from build123d import *

# Parameters (mm, degrees)
PAD_DEPTH       = 1.6
CHAMFER_SIZE    = 0.5
POCKET_DEPTH    = 1.601
PAD018_DEPTH    = 2.5
SKETCH028_R     = 2
POCKET006_DEPTH = 1.6
SKETCH029_R     = 1
POCKET007_DEPTH = 2.501
CHAMFER003_SIZE = 0.95


with BuildPart() as part:
    # Sketch (on Face1 of Binder) → Pad (new body)
    with BuildSketch(Plane.XZ.offset(29.45)):
        with BuildLine():
            Line((-19.5, 11.5), (19.5, 11.5))
            ThreePointArc((21.1, 9.9), (20.631371, 11.031371), (19.5, 11.5))
            Line((21.1, 9.9), (21.1, -1.6))
            ThreePointArc((19.5, -3.2), (20.631371, -2.731371), (21.1, -1.6))
            Line((-19.5, -3.2), (19.5, -3.2))
            ThreePointArc((-21.1, -1.6), (-20.631371, -2.731371), (-19.5, -3.2))
            Line((-21.1, 9.9), (-21.1, -1.6))
            ThreePointArc((-19.5, 11.5), (-20.631371, 11.031371), (-21.1, 9.9))
        make_face()
    extrude(amount=PAD_DEPTH)

    # Chamfer
    chamfer_edges = [part.edges().sort_by_distance(p)[0] for p in [
        (0, -31.05, 11.5),
    ]]
    chamfer(chamfer_edges, length=CHAMFER_SIZE)

    # Sketch023 (on Face4 of Chamfer) → Pocket (cut, through all)
    with BuildSketch(Plane(origin=(0, -29.45, 0), x_dir=(-1, 0, 0), z_dir=(0, 1, 0))):
        with BuildLine():
            Line((3.53, 9.45), (15.53, 9.45))
            ThreePointArc((17.03, 7.95), (16.59066, 9.01066), (15.53, 9.45))
            Line((17.03, 7.95), (17.03, 3.45))
            ThreePointArc((15.53, 1.95), (16.59066, 2.38934), (17.03, 3.45))
            Line((15.53, 1.95), (3.53, 1.95))
            ThreePointArc((2.03, 3.45), (2.46934, 2.38934), (3.53, 1.95))
            Line((2.03, 3.45), (2.03, 7.95))
            ThreePointArc((3.53, 9.45), (2.46934, 9.01066), (2.03, 7.95))
        make_face()
        with BuildLine():
            ThreePointArc((-15.24, 4.9), (-16.159239, 4.519239), (-16.54, 3.6))
            Line((-16.54, 2.8), (-16.54, 3.6))
            ThreePointArc((-16.54, 2.8), (-16.159239, 1.880761), (-15.24, 1.5))
            Line((-8.64, 1.5), (-15.24, 1.5))
            ThreePointArc((-8.64, 1.5), (-7.720761, 1.880761), (-7.34, 2.8))
            Line((-7.34, 3.6), (-7.34, 2.8))
            ThreePointArc((-7.34, 3.6), (-7.720761, 4.519239), (-8.64, 4.9))
            Line((-15.24, 4.9), (-8.64, 4.9))
        make_face()
    extrude(amount=-POCKET_DEPTH, mode=Mode.SUBTRACT)

    # Sketch024 (on Face1 of Binder) → Pad018 (join)
    with BuildSketch(Plane.XZ.offset(29.45)):
        with BuildLine():
            Line((-1, 9.9), (18.5, 9.9))
            ThreePointArc((19.5, 8.9), (19.207107, 9.607107), (18.5, 9.9))
            Line((19.5, 8.9), (19.5, 1.7))
            Line((19.5, 1.7), (17, 1.7))
            Line((17, 1.7), (17, 4.5))
            ThreePointArc((17, 4.5), (16.707107, 5.207107), (16, 5.5))
            Line((16, 5.5), (7.5, 5.5))
            ThreePointArc((7.5, 5.5), (6.792893, 5.207107), (6.5, 4.5))
            Line((6.5, 4.5), (6.5, 2.7))
            ThreePointArc((5.5, 1.7), (6.207107, 1.992893), (6.5, 2.7))
            Line((5.5, 1.7), (-1, 1.7))
            ThreePointArc((-2, 2.7), (-1.707107, 1.992893), (-1, 1.7))
            Line((-2, 2.7), (-2, 8.9))
            ThreePointArc((-1, 9.9), (-1.707107, 9.607107), (-2, 8.9))
        make_face()
        with BuildLine():
            Line((-19.5, -0.1), (7, -0.1))
            Line((7, -0.1), (7, -0.9))
            Line((7, -0.9), (17, -0.9))
            Line((17, -0.9), (17, -0.1))
            Line((17, -0.1), (19.5, -0.1))
            Line((19.5, -0.1), (19.5, -0.6))
            ThreePointArc((18.5, -1.6), (19.207107, -1.307107), (19.5, -0.6))
            Line((18.5, -1.6), (-18.5, -1.6))
            ThreePointArc((-19.5, -0.6), (-19.207107, -1.307107), (-18.5, -1.6))
            Line((-19.5, -0.6), (-19.5, -0.1))
        make_face()
        with BuildLine():
            Line((-18.5, 9.9), (-17.3, 9.9))
            Line((-17.3, 9.9), (-17.3, 1.7))
            Line((-17.3, 1.7), (-19.5, 1.7))
            Line((-19.5, 1.7), (-19.5, 8.9))
            ThreePointArc((-18.5, 9.9), (-19.207107, 9.607107), (-19.5, 8.9))
        make_face()
    extrude(amount=-PAD018_DEPTH)

    # Sketch028 (on Face9 of Pad018) → Pocket006 (cut)
    with BuildSketch(Plane.XZ.offset(31.05)):
        with Locations((2, 7.6)):
            Circle(SKETCH028_R)
    extrude(amount=-POCKET006_DEPTH, mode=Mode.SUBTRACT)

    # Sketch029 (on Face68 of Pocket006) → Pocket007 (cut, through all)
    with BuildSketch(Plane.XZ.offset(29.45)):
        with Locations((2, 7.6)):
            Circle(SKETCH029_R)
    extrude(amount=-POCKET007_DEPTH, mode=Mode.SUBTRACT)

    # Chamfer003
    chamfer003_edges = [part.edges().sort_by_distance(p)[0] for p in [
        (1, -29.45, 7.6),
    ]]
    chamfer(chamfer003_edges, length=CHAMFER003_SIZE)


solid = part.part
Build history of the part. All positions in model axes, mm. A direction names the side the tool comes from. Round coordinates to 2 decimals unless told otherwise and drop trailing zeros. Write each loop counter-clockwise with the first axis right and the second up, starting at its lowest first coordinate (ties: lowest second). Pieces come first, ordered by that corner, then holes. Notation, with made-up numbers: (28.25, 58.25) -> (51.25, 58.25) arc R24 cw to (51.25, 85.25) -> close; hole circle Ø6 at (-16, 57). An arc over 180 degrees is marked (long way). Use one line per item in the form item = value.
Q1. Drop flat-ended pins along their axis: P1, Ø0.8, axis at x = -4, y = -28.5, coming from the +Z side; P2, Ø0.9, axis at y = -28, z = -0.5, coming from the +X side; P3, Ø2, axis at y = -28, z = 6, coming from the -X side. Give the stop position or say it passes through.
Conclusion:
P1 = -0.1
P2 = 19.5
P3 = -19.5
Q2. Tool access for faces 4 (the cylindrical face through (-1.715, -28.218, 2.001)), 5 (the cylindrical face through (1.74, -30.261, 9.583)), 6 (the flat face through (-2.03, -30, 6)), 7 (the cylindrical face through (19.215, -28.218, 9.599)): list every direction of +Z, -Z, +X, -X, +Y, -Y with a clear straight run to the whole face (end or side of a thin tool).
Conclusion:
face_4 = +Y
face_5 = -Y
face_6 = +Y, -Y
face_7 = +Z, +X, +Y
Q3. Band-saw the part on B-B, the plane x = 10.5. Write the cut outline in (y, z), then the cut area to 3 significant figures.
Conclusion:
outline = (-31.05, -2.7) -> (-30.55, -3.2) -> (-29.45, -3.2) -> (-29.45, -1.6) -> (-26.95, -1.6) -> (-26.95, -0.9) -> (-29.45, -0.9) -> (-29.45, 1.5) -> (-31.05, 1.5) -> close; (-31.05, 4.9) -> (-29.45, 4.9) -> (-29.45, 5.5) -> (-26.95, 5.5) -> (-26.95, 9.9) -> (-29.45, 9.9) -> (-29.45, 11.5) -> (-30.55, 11.5) -> (-31.05, 11) -> close
area = 30.6 mm²
Q4. Two-plate mould, pull along Z, no slides. Class faces 1 (the flat face through (12, -30, 4.9)), 2 (the cylindrical face through (19.199, -28.218, -1.315)), 3 (the cylindrical face through (20.64, -29.99, 11.02)): released by +Z, released by -Z, zero draft, split by the parting line, or undercut.
Conclusion:
face_1 = undercut
face_2 = released by -Z
face_3 = released by +Z
Q5. Drill centre lines: L1, parallel to X at y = -30.2, z = 3.75; L2, parallel to Z at x = 2, y = -28; L3, parallel to Z at x = 13.5, y = -27.95. Where is each one in solid material? Low to high.
Conclusion:
L1 = -21.1 to -17.03, -2.03 to 7.35, 16.53 to 21.1
L2 = -1.6 to -0.1, 1.7 to 6.6, 8.6 to 9.9
L3 = -1.6 to -0.9, 5.5 to 9.9
Q6. Band-saw the part on C-C, the plane y = -29.85. Write the cut outline in (x, z), then the cut area to 3 significant figures.
Conclusion:
outline = (-21.1, -1.6) arc R1.6 ccw to (-19.5, -3.2) -> (19.5, -3.2) arc R1.6 ccw to (21.1, -1.6) -> (21.1, 9.9) arc R1.6 ccw to (19.5, 11.5) -> (-19.5, 11.5) arc R1.6 ccw to (-21.1, 9.9) -> close; hole (-17.03, 3.45) arc R1.5 ccw to (-15.53, 1.95) -> (-3.53, 1.95) arc R1.5 ccw to (-2.03, 3.45) -> (-2.03, 7.95) arc R1.5 ccw to (-3.53, 9.45) -> (-15.53, 9.45) arc R1.5 ccw to (-17.03, 7.95) -> close; hole circle Ø4 at (2, 7.6); hole (7.34, 2.8) arc R1.3 ccw to (8.64, 1.5) -> (15.24, 1.5) arc R1.3 ccw to (16.54, 2.8) -> (16.54, 3.6) arc R1.3 ccw to (15.24, 4.9) -> (8.64, 4.9) arc R1.3 ccw to (7.34, 3.6) -> close
area = 465 mm²
Q7. Band-saw the part on A-A, the plane y = -27.85. State how many separate pieces and enclosed holes the cut face has, then the cut area to 3 significant figures.
Conclusion:
separate_pieces = 3
enclosed_holes = 1
area = 201 mm²
Q8. Band-saw the part on D-D, the plane z = 1. Write the cut outline in (x, y).
Conclusion:
outline = (-21.1, -30.55) -> (-20.6, -31.05) -> (20.6, -31.05) -> (21.1, -30.55) -> (21.1, -29.45) -> (-21.1, -29.45) -> close
